```python
from build123d import *

# Parameters (mm, degrees)
SKETCH1_W           = 85.852
SKETCH1_H           = 210.058
BOSS_EXTRUDE1_DEPTH = 6.35
CUT_EXTRUDE1_REACH  = 115.64
SKETCH2_W           = 17.526
SKETCH2_H           = 101.6
SKETCH2_W_2         = 17.653


with BuildPart() as part:
    # Sketch1 → Boss-Extrude1 (new body)
    with BuildSketch(Plane.XY):
        Rectangle(SKETCH1_W, SKETCH1_H)
    extrude(amount=BOSS_EXTRUDE1_DEPTH)

    # Sketch2 → Cut-Extrude1 (cut, up to next)
    with BuildSketch(Plane.XY.offset(6.35), mode=Mode.PRIVATE) as cut_extrude1_sk1:
        with Locations((34.163, -54.229)):
            Rectangle(SKETCH2_W, SKETCH2_H)
    cut_extrude1_tool1 = extrude(cut_extrude1_sk1.sketch, amount=-CUT_EXTRUDE1_REACH, mode=Mode.PRIVATE) & part.part
    # Sketch2 → Cut-Extrude1 (cut, up to next)
    with BuildSketch(Plane.XY.offset(6.35), mode=Mode.PRIVATE) as cut_extrude1_sk2:
        with Locations((-34.0995, -54.229)):
            Rectangle(SKETCH2_W_2, SKETCH2_H)
    cut_extrude1_tool2 = extrude(cut_extrude1_sk2.sketch, amount=-CUT_EXTRUDE1_REACH, mode=Mode.PRIVATE) & part.part
    add(cut_extrude1_tool1.solids().sort_by_distance((34.163, -54.229, 6.35))[0], mode=Mode.SUBTRACT)
    add(cut_extrude1_tool2.solids().sort_by_distance((-34.0995, -54.229, 6.35))[0], mode=Mode.SUBTRACT)


solid = part.part
```
Source: CAD feature listing. Evaluate the final solid. Frame: model axes, mm. A direction names the side the tool comes from. Give positions to 0.01 mm unless a question says otherwise; leave off trailing zeros. Write each loop counter-clockwise with the first axis right and the second up, starting at its lowest first coordinate (ties: lowest second). Pieces come first, ordered by that corner, then holes.
1. Section query A-A (z = 5.25). Return the cut outline in (x, y), then the cut area to 3 significant figures.
2. Section query C-C (y = -43). Return the cut outline in (x, z), then the cut area to 3 significant figures.
3. Section query B-B (x = 27.5). Return the cut outline in (y, z).
4. Access query for faces 1 (the face through (25.4, -55, 3)), 2 (the face through (-1, 25, 6.35)), 3 (the face through (-25.273, -55, 3)). Directions: +Z, -Z, +X, -X, +Y, -Y. A direction counts if a zero-diameter tool reaches every point of the face in a straight line with its end or side. Return the directions, or none.
5. First-contact query: pin 1 (1 mm diameter, centred on x = -27, z = 5, fed in from -Y). Flat tip, straight axial feed; report the tip coordinate or a pass-through.
6. Material intervals for line 1 along X through (y, z) = (-39, 4); line 2 along Y through (x, z) = (-37, 2.75), sorted ascending.
Output values:
1. outline: (-42.93, -3.43) - (-25.27, -3.43) - (-25.27, -105.03) - (25.4, -105.03) - (25.4, -3.43) - (42.93, -3.43) - (42.93, 105.03) - (-42.93, 105.03) - close
1. area: 14,500 mm2
2. outline: (-25.27, 0) - (25.4, 0) - (25.4, 6.35) - (-25.27, 6.35) - close
2. area: 322 mm2
3. outline: (-3.43, 0) - (105.03, 0) - (105.03, 6.35) - (-3.43, 6.35) - close
4. face 1: +Z, -Z, +X, -Y
4. face 2: +Z, +X, -X, +Y, -Y
4. face 3: +Z, -Z, -X, -Y
5. pin 1: stops at y = -3.43
6. line 1: x = -25.27 to 25.4
6. line 2: y = -3.43 to 105.03
